from build123d import *

# Parameters (mm, degrees)
SKETCH1_W           = 31
SKETCH1_H           = 85
BOSS_EXTRUDE1_DEPTH = 7
SKETCH2_R           = 11
CUT_EXTRUDE1_DEPTH  = 100
SKETCH3_R           = 11
CUT_EXTRUDE2_DEPTH  = 7
SKETCH4_W           = 31
SKETCH4_H           = 7.57
BOSS_EXTRUDE3_DEPTH = 25
SKETCH5_R           = 2
CUT_EXTRUDE3_DEPTH  = 14
SKETCH6_R           = 2
CUT_EXTRUDE4_DEPTH  = 14
SKETCH10_W          = 31
SKETCH10_H          = 5
BOSS_EXTRUDE4_DEPTH = 27
SKETCH11_W          = 31
SKETCH11_H          = 6
BOSS_EXTRUDE5_DEPTH = 40
SKETCH9_R           = 8
CUT_EXTRUDE5_DEPTH  = 40
SKETCH13_R          = 4
CUT_EXTRUDE6_DEPTH  = 2
SKETCH15_W          = 7.132198052
SKETCH15_H          = 11.047195358
SKETCH15_W_2        = 7.735251328
SKETCH15_H_2        = 9.356853031
CUT_EXTRUDE9_DEPTH  = 2
CUT_EXTRUDE10_DEPTH = 3


with BuildPart() as part:
    # Sketch1 → Boss-Extrude1 (new body)
    with BuildSketch(Plane(origin=(0, 0, 0), x_dir=(1, 0, 0), z_dir=(0, 1, 0))):
        with Locations((-34.66194332, -13.734817814)):
            Rectangle(SKETCH1_W, SKETCH1_H)
    extrude(amount=BOSS_EXTRUDE1_DEPTH)

    # Sketch2 → Cut-Extrude1 (cut)
    with BuildSketch(Plane(origin=(0, 7, 0), x_dir=(1, 0, 0), z_dir=(0, 1, 0))):
        with Locations(Location((-33.16194332, 0.765182186, 0), (0, 0, 270))):
            Circle(SKETCH2_R)
    extrude(amount=-CUT_EXTRUDE1_DEPTH, mode=Mode.SUBTRACT)

    # Sketch3 → Cut-Extrude2 (cut)
    with BuildSketch(Plane(origin=(0, 7, 0), x_dir=(1, 0, 0), z_dir=(0, 1, 0))):
        with Locations(Location((-33.16194332, -28.434817814, 0), (0, 0, 270))):
            Circle(SKETCH3_R)
    extrude(amount=-CUT_EXTRUDE2_DEPTH, mode=Mode.SUBTRACT)

    # Sketch4 → Boss-Extrude3 (add)
    with BuildSketch(Plane(origin=(0, 7, 0), x_dir=(1, 0, 0), z_dir=(0, 1, 0))):
        with Locations((-34.66194332, -52.449817814)):
            Rectangle(SKETCH4_W, SKETCH4_H)
    extrude(amount=BOSS_EXTRUDE3_DEPTH)

    # Sketch5 → Cut-Extrude3 (cut)
    with BuildSketch(Plane(origin=(0, 0, 48.664817814), x_dir=(-1, 0, 0), z_dir=(0, 0, -1))):
        with Locations((42.16194332, 20)):
            Circle(SKETCH5_R)
        with Locations((27.16194332, 20)):
            Circle(SKETCH5_R)
    extrude(amount=-CUT_EXTRUDE3_DEPTH, mode=Mode.SUBTRACT)

    # Sketch6 → Cut-Extrude4 (cut)
    with BuildSketch(Plane(origin=(0, 7, 0), x_dir=(1, 0, 0), z_dir=(0, 1, 0))):
        with Locations(Location((-43.66194332, -14.434817814, 0), (0, 0, 270))):
            Circle(SKETCH6_R)
        with Locations(Location((-43.66194332, -42.434817814, 0), (0, 0, 270))):
            Circle(SKETCH6_R)
    extrude(amount=-CUT_EXTRUDE4_DEPTH, mode=Mode.SUBTRACT)

    # Sketch10 → Boss-Extrude4 (add)
    with BuildSketch(Plane.XZ):
        with Locations((-34.66194332, -26.265182186)):
            Rectangle(SKETCH10_W, SKETCH10_H)
    extrude(amount=BOSS_EXTRUDE4_DEPTH)

    # Sketch11 → Boss-Extrude5 (add)
    with BuildSketch(Plane.XY.offset(-23.765182186)):
        with Locations((-34.66194332, -24)):
            Rectangle(SKETCH11_W, SKETCH11_H)
    extrude(amount=BOSS_EXTRUDE5_DEPTH)

    # Sketch9 → Cut-Extrude5 (cut)
    with BuildSketch(Plane(origin=(0, 7, 0), x_dir=(1, 0, 0), z_dir=(0, 1, 0))):
        with Locations(Location((-33.16194332, 0.765182186, 0), (0, 0, 270))):
            Circle(SKETCH9_R)
    extrude(amount=-CUT_EXTRUDE5_DEPTH, mode=Mode.SUBTRACT)

    # Sketch13 → Cut-Extrude6 (cut)
    with BuildSketch(Plane(origin=(0, 7, 0), x_dir=(1, 0, 0), z_dir=(0, 1, 0))):
        with Locations(Location((-43.66194332, -14.434817814, 0), (0, 0, 270))):
            Circle(SKETCH13_R)
        with Locations(Location((-43.66194332, -42.434817814, 0), (0, 0, 270))):
            Circle(SKETCH13_R)
    extrude(amount=-CUT_EXTRUDE6_DEPTH, mode=Mode.SUBTRACT)

    # Sketch15 → Cut-Extrude9 (cut)
    with BuildSketch(Plane(origin=(0, 7, 0), x_dir=(1, 0, 0), z_dir=(0, 1, 0))):
        with Locations((-46.595844294, -12.860944888)):
            Rectangle(SKETCH15_W, SKETCH15_H)
        with Locations((-46.294317656, -43.986391299)):
            Rectangle(SKETCH15_W_2, SKETCH15_H_2)
    extrude(amount=-CUT_EXTRUDE9_DEPTH, mode=Mode.SUBTRACT)

    # Sketch17 → Cut-Extrude10 (cut)
    with BuildSketch(Plane(origin=(0, 7, 0), x_dir=(1, 0, 0), z_dir=(0, 1, 0))):
        with BuildLine():
            ThreePointArc((-19.16194332, -18.72671857), (-21.66194332, -22.434817814), (-19.16194332, -26.142917057))
            Line((-19.16194332, -26.142917057), (-19.16194332, -18.72671857))
        make_face()
        with BuildLine():
            Line((-19.16194332, -38.142917057), (-19.16194332, -30.72671857))
            ThreePointArc((-19.16194332, -30.72671857), (-21.66194332, -34.434817814), (-19.16194332, -38.142917057))
        make_face()
    extrude(amount=-CUT_EXTRUDE10_DEPTH, mode=Mode.SUBTRACT)


solid = part.part
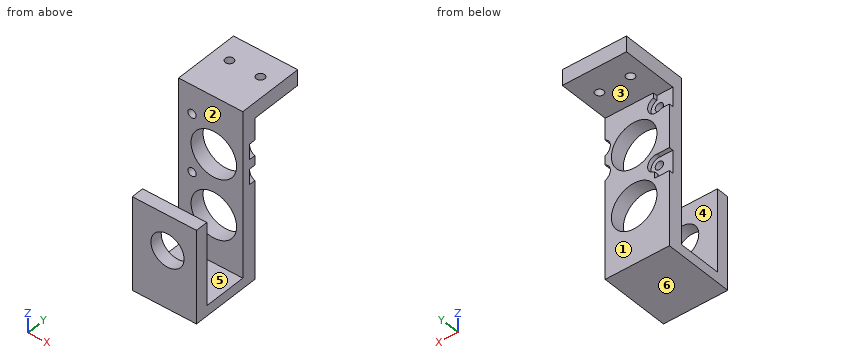
CAD build for the part. Positions are in the model's coordinates, mm. Face numbers are marked on the shaded views. A direction names the side the tool comes from. Round coordinates to 2 decimals unless told otherwise and drop trailing zeros. Order: outer loops, then holes, each group sorted by start corner. A loop starts at its lowest first (then second) coordinate and runs counter-clockwise, first axis right, second up. Notation, with made-up numbers: (9.5, 27) - (55.5, 27) arc R34 ccw to (55.5, 59) - close; hole circle Ø5 at (23, 38). An arc over 180 degrees is marked (long way). Return JSON: item names as keys, results as strings.
(1) Wall check: probe 1 along Z at (x, y) = (-33, 1); probe 2 along Y at (x, z) = (-48, -9); probe 3 along Z at (x, y) = (-28.5, 9). Give the ranges that are in metal, low to high. Write a range as from..to.
Answer key:
{"probe 1": "z = -28.77..-11.76, 10.23..17.44, 39.43..56.23", "probe 2": "y = -27..-21, 0..7", "probe 3": "z = 48.66..56.23"}
(2) Cut at A-A (y = 20). Give the cut face in (x, z).
Answer key:
{"outline": "(-50.16, 48.66) - (-44.16, 48.66) - (-44.16, 56.23) - (-50.16, 56.23) - close; (-40.16, 48.66) - (-29.16, 48.66) - (-29.16, 56.23) - (-40.16, 56.23) - close; (-25.16, 48.66) - (-19.16, 48.66) - (-19.16, 56.23) - (-25.16, 56.23) - close"}
(3) Tool access for the marked faces 5 and 6: list every direction of +Z, -Z, +X, -X, +Y, -Y with a clear straight run to the whole face (end or side of a thin tool).
Answer key:
{"face 5": "+Z, +X, -X", "face 6": "-Z, +X, -X, +Y, -Y"}
(4) Cut at C-C (x = -26.5). Give the cut face in (y, z), then the cut area to 3 significant figures.
Answer key:
{"outline": "(-27, -28.77) - (7, -28.77) - (7, -9.52) - (0, -9.52) - (0, -23.77) - (-21, -23.77) - (-21, -5.19) - (-27, -5.19) - close; (-27, 3.66) - (-21, 3.66) - (-21, 16.23) - (-27, 16.23) - close; (0, 7.99) - (7, 7.99) - (7, 19.68) - (0, 19.68) - close; (0, 37.19) - (7, 37.19) - (7, 48.66) - (18.11, 48.66) - (18.11, 56.23) - (0, 56.23) - close; (21.89, 48.66) - (32, 48.66) - (32, 56.23) - (21.89, 56.23) - close", "area": "832 mm^2"}
(5) Pull direction Y, two halves, no side cores. Call the marked faces 1, 2, 3 and 4: +Y half, -Y half, draft (parallel to the pull), parting line (faces both ways), or undercut.
Answer key:
{"face 1": "+Y half", "face 2": "undercut", "face 3": "draft", "face 4": "undercut"}
(6) Cut at B-B (z = 43). Give the cut face in (x, y), then the cut area to 3 significant figures.
Answer key:
{"outline": "(-50.16, 0) - (-45.58, 0) - (-45.58, 5) - (-50.16, 5) - close; (-41.74, 0) - (-19.16, 0) - (-19.16, 7) - (-39.7, 7) - (-39.7, 5) - (-41.74, 5) - close", "area": "177 mm^2"}
(7) Pin check, flat tips, straight feed: pin 1 Ø12 at (x, z) = (-27, 35.5) entering from -Y; pin 2 Ø10.5 at (x, y) = (-31.5, -5.5) entering from +Z; pin 3 Ø11.5 at (x, z) = (-47, 41) entering from +Y; pin 4 Ø13 at (x, z) = (-33.16, -0.77) entering from +Y. Stop position of each tip, or through.
Answer key:
{"pin 1": "stops at y = 0", "pin 2": "stops at z = -23.77", "pin 3": "stops at y = 7", "pin 4": "passes through"}
(8) Cut at D-D (x = -31.5). Give the cut face in (y, z), then the cut area to 3 significant figures.
Answer key:
{"outline": "(-27, -28.77) - (7, -28.77) - (7, -11.64) - (0, -11.64) - (0, -23.77) - (-21, -23.77) - (-21, -8.59) - (-27, -8.59) - close; (-27, 7.06) - (-21, 7.06) - (-21, 16.23) - (-27, 16.23) - close; (0, 10.11) - (7, 10.11) - (7, 17.56) - (0, 17.56) - close; (0, 39.31) - (7, 39.31) - (7, 48.66) - (32, 48.66) - (32, 56.23) - (0, 56.23) - close", "area": "761 mm^2"}
